Check sheet for the drawn part. Datum: minimum x, y, z corner. Units: mm. Coordinates: 2 decimals unless noted, no trailing zeros. Write each loop counter-clockwise with the first axis right and the second up, starting at its lowest first coordinate (ties: lowest second). Pieces come first, ordered by that corner, then holes. Notation, with made-up numbers: (68.5, 19.25) -> (126.5, 19.25) arc R20 cw to (126.5, 57.25) -> close; hole circle Ø3 at (25.5, 20.25). An arc over 180 degrees is marked (long way). Answer in a Markdown table with one row per item. Add a question column.
1. Cross-section at B-B on y = 54.5. Record the cut outline in (x, z) (3 decimals).
2. Depth check by flat-ended pin: P1, Ø1, axis at x = 53.5, z = 91.5, coming from the -Y side (3 decimals); P2, Ø2, axis at x = 98, z = 99.5, coming from the +Y side; P3, Ø10, axis at x = 69, z = 33.5, coming from the +Y side. Enter the tip coordinate at first touch or a pass-through.
3. Scan lines: L1, parallel to Z at x = 119, y = 64 (1 decimal); L2, parallel to Y at x = 7, z = 13.5 (1 decimal); L3, parallel to Y at x = 78, z = 72 (1 decimal). Record each from-to range of solid material in increasing order. Write a range as from..to.
4. Cross-section at C-C on z = 68. Record the cut outline in (x, y) (3 decimals).
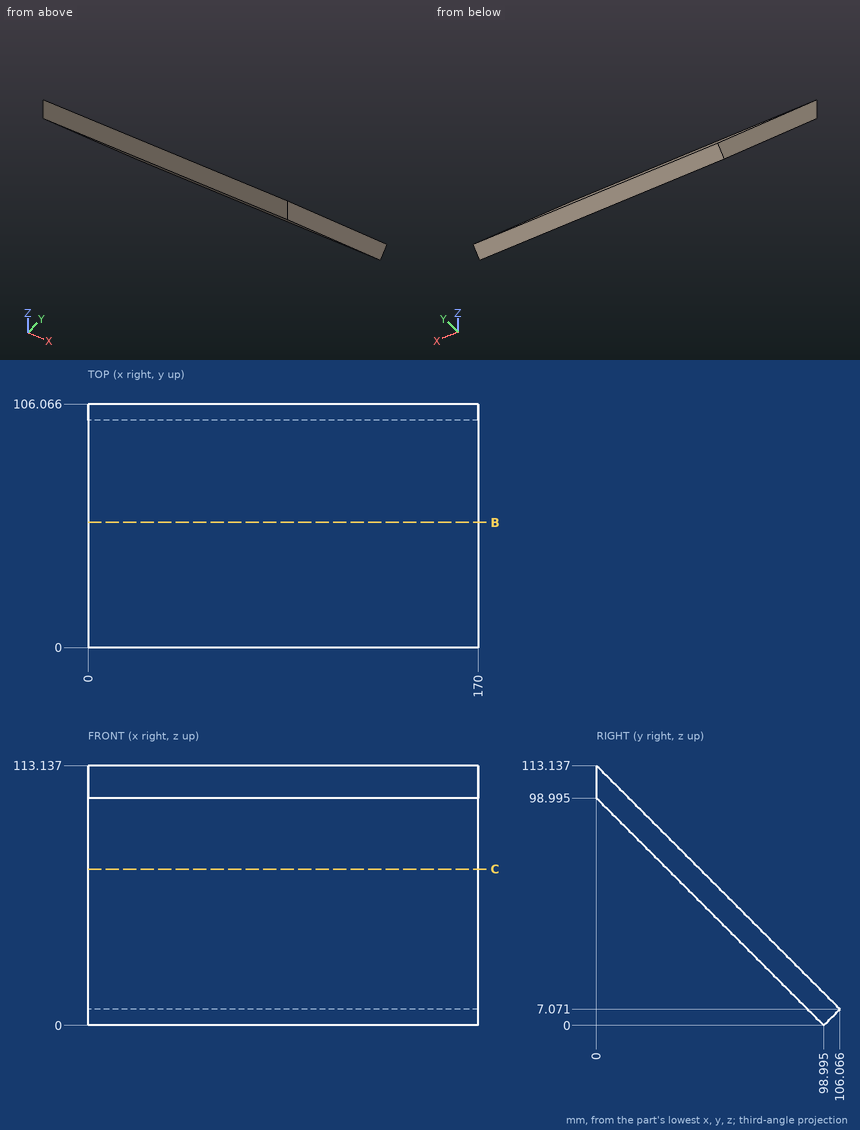
Results found:
| question | item | result |
|---|---|---|
| 1 | outline | (0, 44.495) -> (170, 44.495) -> (170, 58.637) -> (0, 58.637) -> close |
| 2 | P1 | stops at y = 6.995 |
| 2 | P2 | stops at y = 14.64 |
| 2 | P3 | stops at y = 84.64 |
| 3 | L1 | z = 35..49.1 |
| 3 | L2 | y = 85.5..99.6 |
| 3 | L3 | y = 27..41.1 |
| 4 | outline | (0, 30.995) -> (170, 30.995) -> (170, 45.137) -> (0, 45.137) -> close |
